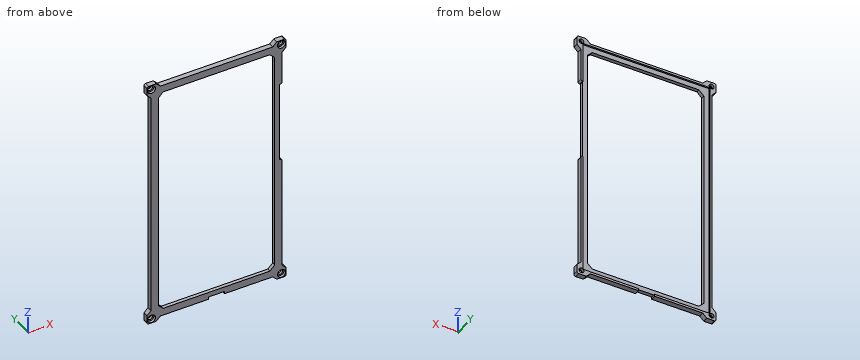
```python
from build123d import *

# Parameters (mm, degrees)
F1_R     = 1.5
F1_W     = 72
F1_H     = 144
F2_DEPTH = 3.175
F3_SIZE  = 3
F4_SIZE  = 2.49999
F5_R     = 1
F6_R     = 2.5
F7_DEPTH = 1.5875
F8_W     = 78.25
F8_H     = 150.25
F9_DEPTH = 1


# Not quite as in the source:
# - a fillet or chamfer is up to 0.001 mm smaller than in the source, because OpenCascade refuses the exact size


with BuildPart() as f2:
    # F1 (on Front) → F2 (new body)
    with BuildSketch(Plane.XZ):
        Polygon((43, 73.2426406871), (43, 79), (37.2426406871, 79), (37.2426406871, 76.5), (-37.2426406871, 76.5), (-37.2426406871, 79), (-43, 79), (-43, 73.2426406871), (-40.5, 73.2426406871), (-40.5, -73.2426406871), (-43, -73.2426406871), (-43, -79), (-37.2426406871, -79), (-37.2426406871, -76.5), (-5, -76.5), (-5, -75), (5, -75), (5, -76.5), (37.2426406871, -76.5), (37.2426406871, -79), (43, -79), (43, -73.2426406871), (40.5, -73.2426406871), (40.5, 0), (39, 0), (39, 50), (40.5, 50), (40.5, 73.2426406871), align=None)
        with Locations((-40.2426406871, -76.2426406871)):
            Circle(F1_R, mode=Mode.SUBTRACT)
        with Locations((40.2426406871, -76.2426406871)):
            Circle(F1_R, mode=Mode.SUBTRACT)
        with Locations((-40.2426406871, 76.2426406871)):
            Circle(F1_R, mode=Mode.SUBTRACT)
        Rectangle(F1_W, F1_H, mode=Mode.SUBTRACT)
        with Locations((40.2426406871, 76.2426406871)):
            Circle(F1_R, mode=Mode.SUBTRACT)
    extrude(amount=F2_DEPTH)

    # F3
    f3_edges = [f2.edges().sort_by_distance(p)[0] for p in [
        (-36, -1.5875, 72),
        (36, -1.5875, 72),
        (36, -1.5875, -72),
        (-36, -1.5875, -72),
    ]]
    chamfer(f3_edges, length=F3_SIZE)

    # F4 (size 2.5 in the source; OpenCascade refuses exactly that, so slightly less here)
    f4_edges = [f2.edges().sort_by_distance(p)[0] for p in [
        (-37.242641, -1.5875, 76.5),
        (-40.5, -1.5875, 73.242641),
        (40.5, -1.5875, 73.242641),
        (37.242641, -1.5875, 76.5),
        (37.242641, -1.5875, -76.5),
        (40.5, -1.5875, -73.242641),
        (-40.5, -1.5875, -73.242641),
        (-37.242641, -1.5875, -76.5),
    ]]
    chamfer(f4_edges, length=F4_SIZE)

    # F5
    f5_edges = [f2.edges().sort_by_distance(p)[0] for p in [
        (-43, -1.5875, 79),
        (43, -1.5875, 79),
        (43, -1.5875, -79),
        (-43, -1.5875, -79),
        (40.5, -1.5875, 0),
        (40.5, -1.5875, 50),
    ]]
    fillet(f5_edges, radius=F5_R)

    # F6 (on face) → F7 (cut)
    with BuildSketch(Plane.XZ.offset(3.175)):
        with Locations((-40.2426406871, 76.2426406871)):
            Circle(F6_R)
        with Locations((40.2426406871, 76.2426406871)):
            Circle(F6_R)
        with Locations((40.2426406871, -76.2426406871)):
            Circle(F6_R)
        with Locations((-40.2426406871, -76.2426406871)):
            Circle(F6_R)
    extrude(amount=-F7_DEPTH, mode=Mode.SUBTRACT)

    # F8 (on face) → F9 (cut)
    with BuildSketch(Plane.XZ):
        Rectangle(F8_W, F8_H)
    extrude(amount=F9_DEPTH, mode=Mode.SUBTRACT)


solid = f2.part
```
Source: CAD feature listing. Evaluate the final solid. Frame: model axes, mm. Give positions to 0.01 mm unless a question says otherwise; leave off trailing zeros. Order: outer loops, then holes, each group sorted by start corner. A loop starts at its lowest first (then second) coordinate and runs counter-clockwise, first axis right, second up.
(1) Section query D-D (y = -2.1). State how many separate pieces and enclosed holes the cut face has, plus the area to 3 significant figures.
(2) Section query C-C (z = 19). Return the cut outline in (x, y) (3 decimals), plus the area to 3 significant figures.
(3) Material intervals for line 1 along Z through (x, y) = (5.5, -1.2); line 2 along X through (y, z) = (-1.7, -36); line 3 along Z through (x, y) = (25, -0.15) (3 decimals), sorted ascending.
(4) Section query B-B (x = -7). Return the cut outline in (y, z) (3 decimals).
(5) Section query A-A (z = -43.5). Return the cut outline in (x, y) (3 decimals), plus the area to 3 significant figures.
(6) Contact query for flat-ended pins moving along their axis: P1, Ø0.8, axis at x = -6.5, y = -0.5, coming from the -Z side; P2, Ø1.5, axis at y = -2.5, z = -2.5, coming from the +X side; P3, Ø0.7, axis at y = -2.5, z = 1.5, coming from the +X side; P4, Ø2.5, axis at x = 40.24, z = 76.24, coming from the -Y side. Output: stop coordinate, or through.
Outcome:
1. separate pieces: 1
1. enclosed holes: 5
1. area: 1,990 mm2
2. outline: (-40.5, -3.175) - (-36, -3.175) - (-36, -1) - (-39.125, -1) - (-39.125, 0) - (-40.5, 0) - close; (36, -3.175) - (39, -3.175) - (39, -1) - (36, -1) - close
2. area: 17.7 mm2
3. line 1: z = -76.5 to -72, 72 to 76.5
3. line 2: x = -40.5 to -36, 36 to 40.5
3. line 3: z = -76.5 to -75.125, 75.125 to 76.5
4. outline: (-3.175, -76.5) - (0, -76.5) - (0, -75.125) - (-1, -75.125) - (-1, -72) - (-3.175, -72) - close; (-3.175, 72) - (-1, 72) - (-1, 75.125) - (0, 75.125) - (0, 76.5) - (-3.175, 76.5) - close
5. outline: (-40.5, -3.175) - (-36, -3.175) - (-36, -1) - (-39.125, -1) - (-39.125, 0) - (-40.5, 0) - close; (36, -3.175) - (40.5, -3.175) - (40.5, 0) - (39.125, 0) - (39.125, -1) - (36, -1) - close
5. area: 22.3 mm2
6. P1: stops at z = -76.5
6. P2: stops at x = 40.5
6. P3: stops at x = 39
6. P4: passes through
